Could you check a few things on this model? Use its own coordinates, in mm. Face numbers are marked on the shaded views. A direction names the side the tool comes from. Give positions to 0.01 mm unless a question says otherwise; leave off trailing zeros. Loops run counter-clockwise (first coordinate to the right, second up) from the corner with the lowest first, then second, coordinate; pieces in that order, holes last.
1. For P1, Ø0.9, axis at y = -8.5, z = -2.5, coming from the -X side; P2, Ø1, axis at x = 8.5, z = 2.5, coming from the -Y side; P3, Ø4.5, axis at y = -2.5, z = -2, coming from the -X side, each with a flat end and sliding along its axis, tell me the tip position at first contact or that it passes through.
2. Imagine slicing it at B-B (y = -26.5). List the corners of the cut face in (x, z) for me, plus the area to 3 significant figures.
3. I need wall thicknesses on line 1 along X through (y, z) = (-22, 2.25); line 2 along X through (y, z) = (-31, 4.75); line 3 along X through (y, z) = (-10, -2.5). Which ranges of each line are inside material? Lowest first, please.
4. Thinking about a two-plate mould opening in Y: for the marked faces 4, 5 and 6, which applies, +Y half, -Y half, draft (parallel to the pull), parting line (faces both ways), or undercut?
5. Imagine slicing it at D-D (x = 0). List the corners of the cut face in (y, z) for me, plus the area to 3 significant figures.
6. For the marked faces 1, 2 and 3, which set-ups out of +Z, -Z, +X, -X, +Y, -Y let a thin tool reach every point of the face, with its end or its side?
7. Imagine slicing it at C-C (x = 13.16). List the corners of the cut face in (y, z) for me, plus the area to 3 significant figures.
8. Imagine slicing it at A-A (z = 1). List the corners of the cut face in (x, y) for me, plus the area to 3 significant figures.
```python
from build123d import *

# Parameters (mm, degrees)
SKETCH1_W           = 46
SKETCH1_H           = 21
SKETCH1_R           = 1.5
BOSS_EXTRUDE1_DEPTH = 3
BOSS_EXTRUDE2_DEPTH = 4
SKETCH5_R           = 8.44
BOSS_EXTRUDE3_DEPTH = 2
FILLET3_R           = 2
CHAMFER1_SIZE       = 0.5


with BuildPart() as part:
    # Sketch1 → Boss-Extrude1 (new body)
    with BuildSketch(Plane.XY):
        with BuildLine():
            Line((19, 0), (-19, 0))
            ThreePointArc((-19, 0), (-23.242640687, -1.757359313), (-25, -6))
            Line((-25, -6), (-25, -33))
            ThreePointArc((-25, -33), (-23.242640687, -37.242640687), (-19, -39))
            Line((-19, -39), (-10.322911411, -39))
            ThreePointArc((-10.322911411, -39), (-6.72058658, -40.201744503), (-4.561286437, -43.325581395))
            ThreePointArc((-4.561286437, -43.325581395), (0, -46.75), (4.561286437, -43.325581395))
            ThreePointArc((4.561286437, -43.325581395), (6.72058658, -40.201744503), (10.322911411, -39))
            Line((10.322911411, -39), (19, -39))
            ThreePointArc((19, -39), (23.242640687, -37.242640687), (25, -33))
            Line((25, -33), (25, -6))
            ThreePointArc((25, -6), (23.242640687, -1.757359313), (19, 0))
        make_face()
        with Locations((0, -26.5)):
            Rectangle(SKETCH1_W, SKETCH1_H, mode=Mode.SUBTRACT)
        with Locations((0, -42)):
            Circle(SKETCH1_R, mode=Mode.SUBTRACT)
        with Locations((-20, -5)):
            Circle(SKETCH1_R, mode=Mode.SUBTRACT)
        with Locations((20, -5)):
            Circle(SKETCH1_R, mode=Mode.SUBTRACT)
    extrude(amount=BOSS_EXTRUDE1_DEPTH)

    # Sketch3 → Boss-Extrude2 (add)
    with BuildSketch(Plane(origin=(0, 0, 0), x_dir=(-1, 0, 0), z_dir=(0, 0, -1))):
        Polygon((-7.223, 0), (-7.223, -5.965393219), (-6.223, -6.965393219), (-6.223, -10.04450176), (6.223, -10.04450176), (6.223, -6.965393219), (7.223, -5.965393219), (7.223, 0), align=None)
    extrude(amount=BOSS_EXTRUDE2_DEPTH)

    # Sketch5 → Boss-Extrude3 (add)
    with BuildSketch(Plane.XY.offset(3)):
        with BuildLine():
            Line((19, 0), (-19, 0))
            ThreePointArc((-19, 0), (-23.242640687, -1.757359313), (-25, -6))
            Line((-25, -6), (-25, -33))
            ThreePointArc((-25, -33), (-23.242640687, -37.242640687), (-19, -39))
            Line((-19, -39), (-10.322911411, -39))
            ThreePointArc((-10.322911411, -39), (-6.72058658, -40.201744503), (-4.561286437, -43.325581395))
            ThreePointArc((-4.561286437, -43.325581395), (0, -46.75), (4.561286437, -43.325581395))
            ThreePointArc((4.561286437, -43.325581395), (6.72058658, -40.201744503), (10.322911411, -39))
            Line((10.322911411, -39), (19, -39))
            ThreePointArc((19, -39), (23.242640687, -37.242640687), (25, -33))
            Line((25, -33), (25, -6))
            ThreePointArc((25, -6), (23.242640687, -1.757359313), (19, 0))
        make_face()
        with Locations((13.16, -26.5)):
            Circle(SKETCH5_R, mode=Mode.SUBTRACT)
        with Locations((-12.34, -26.5)):
            Circle(SKETCH5_R, mode=Mode.SUBTRACT)
    extrude(amount=BOSS_EXTRUDE3_DEPTH)

    # Fillet3
    fillet3_edges = [part.edges().sort_by_distance(p)[0] for p in [
        (-6.72058658, -40.201744503, 5),
        (0, -46.75, 5),
        (6.72058658, -40.201744503, 5),
        (14.661455706, -39, 5),
        (23.242640687, -37.242640687, 5),
        (25, -19.5, 5),
        (23.242640687, -1.757359313, 5),
        (0, 0, 5),
        (-23.242640687, -1.757359313, 5),
        (-25, -19.5, 5),
        (-23.242640687, -37.242640687, 5),
        (-14.661455706, -39, 5),
    ]]
    fillet(fillet3_edges, radius=FILLET3_R)

    # Chamfer1
    chamfer1_edges = [part.edges().sort_by_distance(p)[0] for p in [
        (-20.78, -26.5, 5),
        (4.72, -26.5, 5),
    ]]
    chamfer(chamfer1_edges, length=CHAMFER1_SIZE)


solid = part.part
```
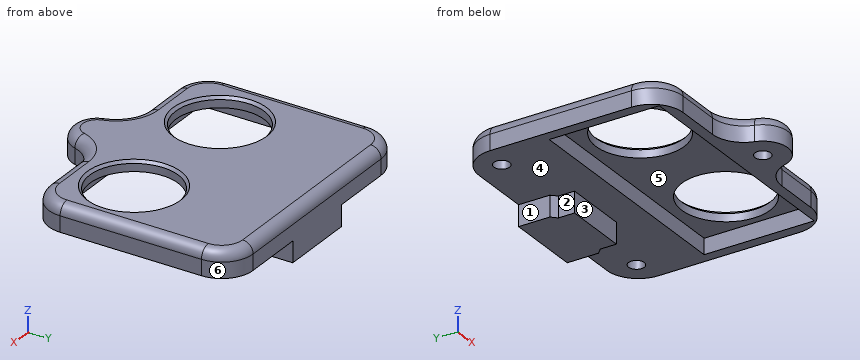
Derived:
1. P1: stops at x = -6.22
1. P2: stops at y = -39.47
1. P3: stops at x = -24.47
2. outline: (-25, 0) - (-23, 0) - (-23, 3) - (-20.78, 3) - (-20.78, 4.5) - (-21.28, 5) - (-23, 5) arc R2 ccw to (-25, 3) - close; (-3.9, 3) - (4.72, 3) - (4.72, 4.5) - (4.22, 5) - (-3.4, 5) - (-3.9, 4.5) - close; (21.6, 3) - (23, 3) - (23, 0) - (25, 0) - (25, 3) arc R2 ccw to (23, 5) - (22.1, 5) - (21.6, 4.5) - close
2. area: 42.3 mm2
3. line 1: x = -25 to -23, 23 to 25
3. line 2: x = -23.97 to -19.77, -4.91 to 5.73, 20.59 to 23.97
3. line 3: x = -6.22 to 6.22
4. face 4: draft
4. face 5: undercut
4. face 6: +Y half
5. outline: (-46.75, 0) - (-43.5, 0) - (-43.5, 3) - (-40.5, 3) - (-40.5, 0) - (-37, 0) - (-37, 3) - (-16, 3) - (-16, 0) - (-10.04, 0) - (-10.04, -4) - (0, -4) - (0, 3) arc R2 ccw to (-2, 5) - (-44.75, 5) arc R2 ccw to (-46.75, 3) - close
5. area: 200 mm2
6. face 1: -Z, -X, +Y, -Y
6. face 2: -Z, -X, -Y
6. face 3: -Z, +X, -X, -Y
7. outline: (-39, 0) - (-37, 0) - (-37, 3) - (-34.94, 3) - (-34.94, 4.5) - (-35.44, 5) - (-37, 5) arc R2 ccw to (-39, 3) - close; (-18.06, 3) - (-16, 3) - (-16, 0) - (0, 0) - (0, 3) arc R2 ccw to (-2, 5) - (-17.56, 5) - (-18.06, 4.5) - close
7. area: 96.3 mm2
8. outline: (-25, -33) arc R6 ccw to (-19, -39) - (-10.32, -39) arc R6 cw to (-4.56, -43.33) arc R4.75 ccw to (4.56, -43.33) arc R6 cw to (10.32, -39) - (19, -39) arc R6 ccw to (25, -33) - (25, -6) arc R6 ccw to (19, 0) - (-19, 0) arc R6 ccw to (-25, -6) - close; hole (-23, -37) - (23, -37) - (23, -16) - (-23, -16) - close; hole circle Ø3 at (-20, -5); hole circle Ø3 at (0, -42); hole circle Ø3 at (20, -5)
8. area: 1,010 mm2
